Answer from the drawing. Dimensions are ordinates in mm from the lowest x, y and z of the part. A direction names the side the tool comes from. Coordinates: 2 decimals unless noted, no trailing zeros. Write each loop counter-clockwise with the first axis right and the second up, starting at its lowest first coordinate (ties: lowest second). Pieces come first, ordered by that corner, then holes.
(1) Given P1, Ø1, axis at x = 4, z = 14, coming from the -Y side; P2, Ø8, axis at x = 8.5, y = 11.5, coming from the -Z side; P3, Ø8, axis at x = 11, z = 10, coming from the -Y side; P4, Ø1, axis at x = 7.5, y = 19.5, coming from the +Z side, each flat-ended and moving along its own axis, determine where each tip first touches the part or whether it passes through.
(2) The part is cut by section C-C on x = 5. Determine the outline of the cut face in (y, z), plus the area to 3 significant figures.
(3) Straight lines are drawn through the part: line 1 (Y direction, x = 7, z = 3.5); line 2 (Z direction, x = 8.75, y = 11) (1 decimal); line 3 (Z direction, x = 8, y = 26.5) (1 decimal). For each, find the intervals that lie inside material, in ascending order.
(4) The part is cut by section B-B on z = 8.5. Determine the outline of the cut face in (x, y).
(5) Which of the six approach directions +Z, -Z, +X, -X, +Y, -Y give full straight-line access (tool end or side, diameter ignored) to the marked faces 1 and 2?
(6) The part is cut by section D-D on z = 5.25. Determine the outline of the cut face in (x, y).
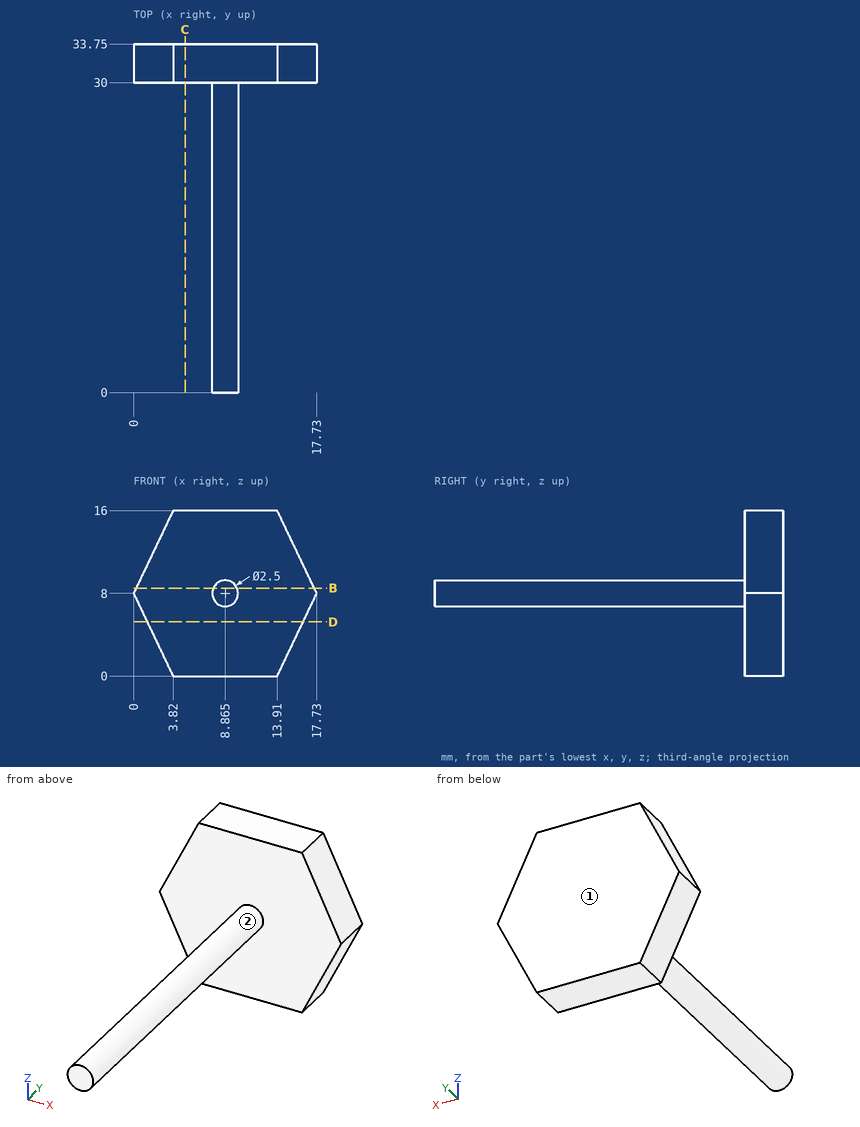
Model answer:
1. P1: stops at y = 30
1. P2: stops at z = 6.75
1. P3: stops at y = 0
1. P4: stops at z = 8.9
2. outline: (30, 0) - (33.75, 0) - (33.75, 16) - (30, 16) - close
2. area: 60.0 mm2
3. line 1: y = 30 to 33.75
3. line 2: z = 6.8 to 9.2
3. line 3: z = 7.1 to 8.9
4. outline: (0.24, 30) - (7.72, 30) - (7.72, 0) - (10.01, 0) - (10.01, 30) - (17.49, 30) - (17.49, 33.75) - (0.24, 33.75) - close
5. face 1: +Z, -Z, +X, -X, +Y
5. face 2: -Y
6. outline: (1.31, 30) - (16.42, 30) - (16.42, 33.75) - (1.31, 33.75) - close
